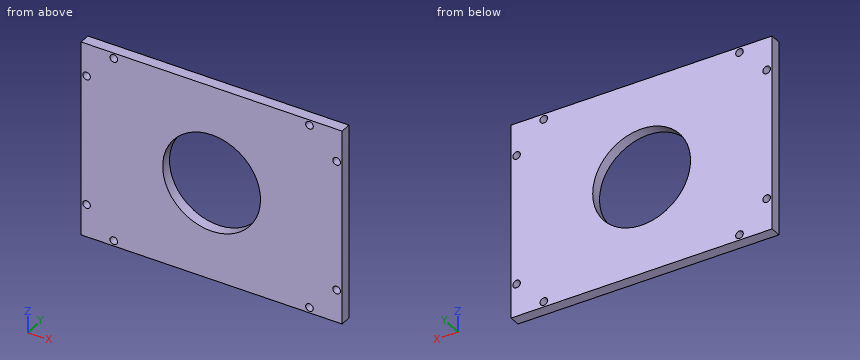
Autodesk Inventor part; units mm, degrees
ref_plane "YZ Plane" through (0, 0, 0) normal (1, 0, 0) x (0, 1, 0)
ref_plane "XZ Plane" through (0, 0, 0) normal (0, 1, 0) x (-1, 0, 0)
ref_plane "XY Plane" through (0, 0, 0) normal (0, 0, 1) x (1, 0, 0)
sketch "Sketch1" plane through (0, 0, 0) normal (0, 1, 0) x (-1, 0, 0)
  line L0 (0, 0) -> (-120, 0)
  line L1 (-120, 0) -> (-120, 90)
  line L2 (-120, 90) -> (0, 90)
  line L3 (0, 90) -> (0, 0)
  line L4 (0, 0) -> (-60, 0)
  line L5 (-60, 0) -> (-60, 45)
  line L6 (-60, 45) -> (0, 45)
  line L7 (0, 45) -> (0, 0)
  circle A0 centre (-60, 45) radius 22.5
  dimension "d0" = 120
  dimension "d1" = 90
  dimension "d2" = 60
  dimension "d3" = 45
  dimension "d4" = 45
extrude "Extrusion1" add sketch "Sketch1" against normal blind 5
sketch "Sketch2" plane through (0, 0, 0) normal (0, 1, 0) x (1, 0, 0)
  line L0 (0, -90) -> (0, 0)
  line L1 (0, 0) -> (60, 0)
  line L2 (60, 0) -> (60, -45)
  line L3 (60, -45) -> (0, -45)
  line L4 (0, -45) -> (0, 0)
  circle A0 centre (60, -45) radius 22.5
  dimension "d7" = 60
  dimension "d8" = 45
  dimension "d9" = 45
extrude "Extrusion2" cut sketch "Sketch2" against normal blind 5 contours A0 L2 L3 | L3 L2 A0
sketch "Sketch3" plane through (0, 0, 0) normal (0, 1, 0) x (1, 0, 0)
  line L0 (0, 0) -> (120, 0)
  line L1 (0, 0) -> (15, 0)
  line L2 (15, 0) -> (15, -2.5)
  line L3 (15, -2.5) -> (0, -2.5)
  line L4 (0, -2.5) -> (0, 0)
  circle A0 centre (15, -2.5) radius 1.75
  dimension "d12" = 15
  dimension "d13" = 2.5
  dimension "d14" = 3.5
extrude "Extrusion3" cut sketch "Sketch3" against normal blind 5 contours A0 L3 L2 | L2 L3 A0
sketch "Sketch4" plane through (0, 0, 0) normal (0, 1, 0) x (1, 0, 0)
  line L0 (120, -90) -> (0, -90)
  line L1 (0, -90) -> (15, -90)
  line L2 (15, -90) -> (15, -87.5)
  line L3 (15, -87.5) -> (0, -87.5)
  line L4 (0, -87.5) -> (0, -90)
  circle A0 centre (15, -87.5) radius 1.75
  point P0 (0, 0)
  dimension "d17" = 15
  dimension "d18" = 2.5
  dimension "d19" = 3.5
extrude "Extrusion4" cut sketch "Sketch4" against normal blind 5 contours A0 L3 L2 | L2 L3 A0
sketch "Sketch5" plane through (0, 0, 0) normal (0, 1, 0) x (1, 0, 0)
  line L0 (120, 0) -> (120, -90)
  line L1 (120, 0) -> (105, 0)
  line L2 (105, 0) -> (105, -2.5)
  line L3 (105, -2.5) -> (120, -2.5)
  line L4 (120, -2.5) -> (120, 0)
  circle A0 centre (105, -2.5) radius 1.75
  point P0 (0, 0)
  dimension "d22" = 15
  dimension "d23" = 2.5
  dimension "d32" = 3.5
extrude "Extrusion5" [suppressed]
sketch "Sketch6" plane through (0, 0, 0) normal (0, 1, 0) x (1, 0, 0)
  line L0 (120, 0) -> (120, -90)
  line L1 (120, -90) -> (105, -90)
  line L2 (105, -90) -> (105, -87.5)
  line L3 (105, -87.5) -> (120, -87.5)
  line L4 (120, -87.5) -> (120, -90)
  circle A0 centre (105, -87.5) radius 1.75
  point P0 (0, 0)
  dimension "d27" = 15
  dimension "d28" = 2.5
  dimension "d29" = 3.5
extrude "Extrusion6" cut sketch "Sketch6" against normal blind 5 contours A0 L2 L3 | L3 L2 A0
sketch "Sketch7" plane through (0, 0, 0) normal (0, 1, 0) x (1, 0, 0)
  line L0 (0, 0) -> (120, 0)
  line L1 (120, 0) -> (105, 0)
  line L2 (105, 0) -> (105, -2.5)
  line L3 (105, -2.5) -> (120, -2.5)
  line L4 (120, -2.5) -> (120, 0)
  circle A0 centre (105, -2.5) radius 1.75
  dimension "d33" = 15
  dimension "d34" = 2.5
  dimension "d35" = 3.5
extrude "Extrusion7" cut sketch "Sketch7" against normal blind 5 contours A0 L3 L2 | L2 L3 A0
sketch "Sketch8" plane through (0, 0, 0) normal (0, 1, 0) x (1, 0, 0)
  line L0 (0, 0) -> (2.5, 0)
  line L1 (2.5, 0) -> (2.5, -15)
  line L2 (2.5, -15) -> (0, -15)
  line L3 (0, -15) -> (0, 0)
  circle A0 centre (2.5, -15) radius 1.75
  dimension "d38" = 2.5
  dimension "d39" = 15
  dimension "d40" = 3.5
extrude "Extrusion8" cut sketch "Sketch8" against normal blind 10 contours A0 L2 L1 | L1 L2 A0
sketch "Sketch9" plane through (0, 0, 0) normal (0, 1, 0) x (1, 0, 0)
  line L0 (0, -90) -> (2.5, -90)
  line L1 (2.5, -90) -> (2.5, -75)
  line L2 (2.5, -75) -> (0, -75)
  line L3 (0, -75) -> (0, -90)
  circle A0 centre (2.5, -75) radius 1.75
  point P0 (0, 0)
  dimension "d43" = 2.5
  dimension "d44" = 15
  dimension "d45" = 3.5
extrude "Extrusion9" cut sketch "Sketch9" against normal blind 10 contours A0 L2 L1 | L1 L2 A0
sketch "Sketch10" plane through (0, 0, 0) normal (0, 1, 0) x (1, 0, 0)
  line L0 (120, 0) -> (120, -90)
  point P0 (0, 0)
sketch "Sketch11" plane through (0, 0, 0) normal (0, 1, 0) x (1, 0, 0)
  line L0 (120, 0) -> (120, -90)
  line L1 (120, 0) -> (117.5, 0)
  line L2 (117.5, 0) -> (117.5, -15)
  line L3 (117.5, -15) -> (120, -15)
  line L4 (120, -15) -> (120, 0)
  circle A0 centre (117.5, -15) radius 1.75
  point P0 (0, 0)
  dimension "d50" = 2.5
  dimension "d51" = 15
  dimension "d52" = 3.5
extrude "Extrusion10" cut sketch "Sketch11" against normal blind 10 contours A0 L2 L3 | L3 L2 A0
sketch "Sketch12" plane through (0, 0, 0) normal (0, 1, 0) x (1, 0, 0)
  line L0 (120, -90) -> (0, -90)
  line L1 (120, -90) -> (117.5, -90)
  line L2 (117.5, -90) -> (117.5, -75)
  line L3 (117.5, -75) -> (120, -75)
  line L4 (120, -75) -> (120, -90)
  circle A0 centre (117.5, -75) radius 1.75
  point P0 (0, 0)
  dimension "d55" = 2.5
  dimension "d56" = 15
  dimension "d57" = 3.5
extrude "Extrusion11" cut sketch "Sketch12" against normal blind 10 contours A0 L3 L2 | L2 L3 A0
properties part number "expo2"
Work out the finished part from the listing and answer in its coordinate system (mm). Give positions to 0.01 mm unless a question says otherwise; leave off trailing zeros. Loops run counter-clockwise (first coordinate to the right, second up) from the corner with the lowest first, then second, coordinate; pieces in that order, holes last. Notation, with made-up numbers: (35, 10) - (87, 10) arc R28 cw to (87, 43) - close; hole circle Ø4 at (12, -27.75). An arc over 180 degrees is marked (long way). Answer in a Markdown table with one row per item. Add a question column.
Q1. This flat-tipped pin is pushed along its axis until it touches: P1, Ø2, axis at x = 105, z = 2.5, coming from the +Y side. Where does it stop, or does it pass through?
Q2. The part is cut by section D-D (z = 45). Determine the outline of the cut face in (x, y).
Q3. The part is cut by section A-A (z = 87.5). Determine the outline of the cut face in (x, y).
Q4. Consider line 1 along Z through (x, y) = (117.5, -2.65); line 2 along Z through (x, y) = (105, -3.35); line 3 along X through (y, z) = (-2.4, 87.5). Determine where each line is inside the solid, lowest interval first.
Q5. The part is cut by section B-B (y = -1.25). State how many separate pieces and enclosed holes the cut face has, and give its area (3 significant figures).
Q6. The part is cut by section C-C (x = 117.5). Determine the outline of the cut face in (y, z), and give its area (3 significant figures).
Solution:
| question | item | result |
|---|---|---|
| 1 | P1 | passes through |
| 2 | outline | (0, -5) - (37.5, -5) - (37.5, 0) - (0, 0) - close; (82.5, -5) - (120, -5) - (120, 0) - (82.5, 0) - close |
| 3 | outline | (0, -5) - (13.25, -5) - (13.25, 0) - (0, 0) - close; (16.75, -5) - (103.25, -5) - (103.25, 0) - (16.75, 0) - close; (106.75, -5) - (120, -5) - (120, 0) - (106.75, 0) - close |
| 4 | line 1 | z = 0 to 13.25, 16.75 to 73.25, 76.75 to 90 |
| 4 | line 2 | z = 0 to 0.75, 4.25 to 85.75, 89.25 to 90 |
| 4 | line 3 | x = 0 to 13.25, 16.75 to 103.25, 106.75 to 120 |
| 5 | separate pieces | 1 |
| 5 | enclosed holes | 9 |
| 5 | area | 9,130 mm² |
| 6 | outline | (-5, 0) - (0, 0) - (0, 13.25) - (-5, 13.25) - close; (-5, 16.75) - (0, 16.75) - (0, 73.25) - (-5, 73.25) - close; (-5, 76.75) - (0, 76.75) - (0, 90) - (-5, 90) - close |
| 6 | area | 415 mm² |
